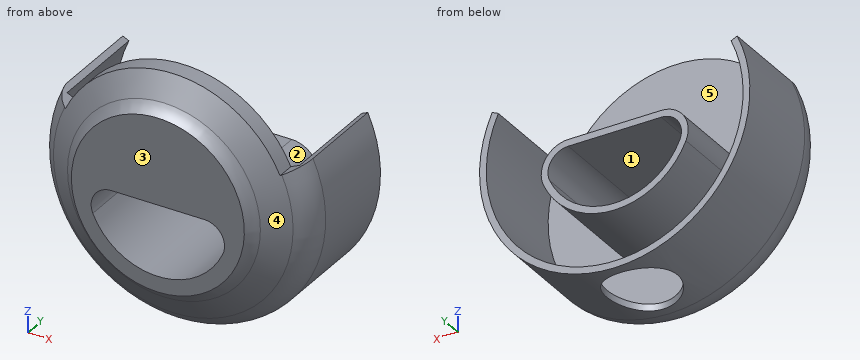
from build123d import *

# Parameters (mm, degrees)
CUT_EXTRUDE3_DEPTH           = 60
CUT_EXTRUDE5_DEPTH           = 2
CUT_EXTRUDE5_DEPTH_BACK      = 30
SKETCH9_R                    = 38
SKETCH9_R_2                  = 23
SKETCH19_W                   = 12
SKETCH19_H                   = 36.5
CUT_REVOLVE2_ANGLE           = 65
CUT_REVOLVE2_OTHER_WAY_ANGLE = 65
SKETCH21_W                   = 3.25
SKETCH21_H                   = 4
BOSS_EXTRUDE3_DEPTH          = 1.35
CIRPATTERN1_COUNT            = 5
CUT_EXTRUDE9_START           = -5
CUT_EXTRUDE9_DEPTH           = 5
SKETCH23_R                   = 10.5
CUT_EXTRUDE10_DEPTH          = 10
SKETCH24_W                   = 15
SKETCH24_H                   = 8
BOSS_EXTRUDE4_DEPTH          = 8
SKETCH26_W                   = 10
SKETCH26_H                   = 6
CUT_EXTRUDE11_DEPTH          = 10
SKETCH27_W                   = 4
SKETCH27_H                   = 5
CUT_EXTRUDE12_DEPTH          = 5
CUT_EXTRUDE14_DEPTH          = 2
CUT_EXTRUDE14_DEPTH_BACK     = 30
SKETCH29_R                   = 1
CUT_EXTRUDE15_DEPTH          = 15
FILLET1_R                    = 6
FILLET2_R                    = 8
INTERSECT2_START             = 55.427876097
INTERSECT2_OUTLINE_W         = 10
INTERSECT2_OUTLINE_H         = 6
INTERSECT2_DEPTH             = 8
INTERSECT2_2_DEPTH           = 13
INTERSECT2_START_2           = 50.427876097
INTERSECT2_3_OUTLINE_W       = 15
INTERSECT2_3_OUTLINE_H       = 8
INTERSECT2_3_OUTLINE_W_2     = 10
INTERSECT2_3_OUTLINE_H_2     = 6
INTERSECT2_3_DEPTH           = 5


# Read off the part's stored shape, not the designer's step: Cut-Extrude9, Intersect2
with BuildPart() as part:
    # Sketch1 → Revolve1 (revolve)
    with BuildSketch(Plane.XY, mode=Mode.PRIVATE) as revolve1_sk:
        with BuildLine():
            Line((0, 63.427876097), (32, 63.427876097))
            ThreePointArc((32, 63.427876097), (37.656854249, 61.084730346), (40, 55.427876097))
            Line((40, 55.427876097), (40, 28.846818009))
            ThreePointArc((40, 28.846818009), (38.792081772, 24.082439968), (35.460140376, 20.469057744))
            Line((35.460140376, 20.469057744), (28.539859624, 15.958818353))
            ThreePointArc((28.539859624, 15.958818353), (25.207918228, 12.345436129), (24, 7.581058088))
            Line((24, 7.581058088), (24, 3.25))
            Line((24, 3.25), (24.35, 3))
            Line((24.35, 3), (24.35, 0))
            Line((24.35, 0), (22.5, 0))
            Line((22.5, 0), (22.5, 12.5))
            ThreePointArc((22.5, 12.5), (22.353553391, 12.853553391), (22, 13))
            Line((22, 13), (0, 13))
            Line((0, 13), (0, 63.427876097))
        make_face()
    revolve(revolve1_sk.sketch.rotate(Axis((0, 0, 0), (0, 1, 0)), 90), axis=Axis((0, 0, 0), (0, 1, 0)))

    # Sketch11 → Cut-Extrude3 (cut)
    with BuildSketch(Plane(origin=(0, 13, 0), x_dir=(-1, 0, 0), z_dir=(0, -1, 0))):
        with BuildLine():
            Line((-21, 0), (21, 0))
            ThreePointArc((21, 0), (0, 21), (-21, 0))
        make_face()
    extrude(amount=-CUT_EXTRUDE3_DEPTH, mode=Mode.SUBTRACT)

    # Sketch9 → Cut-Extrude5 (cut, two sides: drawn at the far end of the back side and taken through both)
    with BuildSketch(Plane(origin=(0, 55.427876097, 0), x_dir=(1, 0, 0), z_dir=(0, 1, 0)).offset(-CUT_EXTRUDE5_DEPTH_BACK)):
        with Locations(Location((0, 0, 0), (0, 0, 270))):
            Circle(SKETCH9_R)
        with Locations(Location((0, 0, 0), (0, 0, 270))):
            Circle(SKETCH9_R_2, mode=Mode.SUBTRACT)
    extrude(amount=CUT_EXTRUDE5_DEPTH + CUT_EXTRUDE5_DEPTH_BACK, mode=Mode.SUBTRACT)

    # Sketch19 → Cut-Revolve2 (revolve, cut)
    with BuildSketch(Plane(origin=(0, 0, 0), x_dir=(0, 0, -1), z_dir=(1, 0, 0))):
        with Locations((-41.064715832, 37.177876097)):
            Rectangle(SKETCH19_W, SKETCH19_H)
    revolve(axis=Axis((0, 0, 0), (0, 1, 0)), revolution_arc=CUT_REVOLVE2_ANGLE, mode=Mode.SUBTRACT)

    # Sketch19 → Cut-Revolve2 other way (revolve, cut)
    with BuildSketch(Plane(origin=(0, 0, 0), x_dir=(0, 0, -1), z_dir=(1, 0, 0))):
        with Locations((-41.064715832, 37.177876097)):
            Rectangle(SKETCH19_W, SKETCH19_H)
    revolve(axis=Axis((0, 0, 0), (0, -1, 0)), revolution_arc=CUT_REVOLVE2_OTHER_WAY_ANGLE, mode=Mode.SUBTRACT)

    # Sketch21 → Boss-Extrude3 (add)
    with BuildSketch(Plane(origin=(0, 0, 22.5), x_dir=(-1, 0, 0), z_dir=(0, 0, -1))):
        with Locations((0, 2)):
            Rectangle(SKETCH21_W, SKETCH21_H)
    boss_extrude3 = extrude(amount=BOSS_EXTRUDE3_DEPTH)

    # CirPattern1: Boss-Extrude3 ×5 about axis
    cirpattern1_axis = Axis((0, 0, 0), (0, 1, 0))
    for i in range(1, CIRPATTERN1_COUNT):
        add(boss_extrude3.rotate(cirpattern1_axis, i * 360 / CIRPATTERN1_COUNT))

    # Cut-Extrude9 outline → Cut-Extrude9 (cut)
    with BuildSketch(Plane(origin=(0, 63.427876097, 0), x_dir=(1, 0, 0), z_dir=(0, 1, 0)).offset(CUT_EXTRUDE9_START)):
        with BuildLine():
            ThreePointArc((40, 0), (0, 40), (-40, 0))
            Line((-40, 0), (-21, 0))
            ThreePointArc((-21, 0), (0, 21), (21, 0))
            Line((21, 0), (40, 0))
        make_face()
    extrude(amount=CUT_EXTRUDE9_DEPTH, mode=Mode.SUBTRACT)

    # Sketch23 → Cut-Extrude10 (cut)
    with BuildSketch(Plane(origin=(0, 0, -40), x_dir=(-1, 0, 0), z_dir=(0, 0, -1))):
        with Locations((0, 42.137876097)):
            Circle(SKETCH23_R)
    extrude(amount=-CUT_EXTRUDE10_DEPTH, mode=Mode.SUBTRACT)

    # Sketch24 → Boss-Extrude4 (add)
    with BuildSketch(Plane(origin=(0, 58.427876097, 0), x_dir=(1, 0, 0), z_dir=(0, 1, 0))):
        with Locations((0, 30)):
            Rectangle(SKETCH24_W, SKETCH24_H)
    extrude(amount=-BOSS_EXTRUDE4_DEPTH)

    # Sketch26 → Cut-Extrude11 (cut)
    with BuildSketch(Plane(origin=(0, 58.427876097, 0), x_dir=(1, 0, 0), z_dir=(0, 1, 0))):
        with Locations((0, 30)):
            Rectangle(SKETCH26_W, SKETCH26_H)
    extrude(amount=-CUT_EXTRUDE11_DEPTH, mode=Mode.SUBTRACT)

    # Sketch27 → Cut-Extrude12 (cut)
    with BuildSketch(Plane(origin=(7.5, 0, 0), x_dir=(0, 0, -1), z_dir=(1, 0, 0))):
        with Locations((30, 53.927876097)):
            Rectangle(SKETCH27_W, SKETCH27_H)
    extrude(amount=-CUT_EXTRUDE12_DEPTH, mode=Mode.SUBTRACT)

    # Sketch28 → Cut-Extrude14 (cut, two sides: drawn at the far end of the back side and taken through both)
    with BuildSketch(Plane(origin=(0, 55.427876097, 0), x_dir=(1, 0, 0), z_dir=(0, 1, 0)).offset(-CUT_EXTRUDE14_DEPTH_BACK)):
        with BuildLine():
            Line((-22.912878475, -2), (22.912878475, -2))
            ThreePointArc((22.912878475, -2), (0, -23), (-22.912878475, -2))
        make_face()
    extrude(amount=CUT_EXTRUDE14_DEPTH + CUT_EXTRUDE14_DEPTH_BACK, mode=Mode.SUBTRACT)

    # Sketch29 → Cut-Extrude15 (cut)
    with BuildSketch(Plane(origin=(0, 0, 0), x_dir=(-1, 0, 0), z_dir=(0, 0, -1))):
        with Locations((-30.416198487, 60.927876097)):
            Circle(SKETCH29_R)
        with Locations((30.416198487, 60.927876097)):
            Circle(SKETCH29_R)
        with Locations((0, 60.927876097)):
            Circle(SKETCH29_R)
    extrude(amount=-CUT_EXTRUDE15_DEPTH, mode=Mode.SUBTRACT)

    # Fillet1
    fillet1_edges = [part.edges().sort_by_distance(p)[0] for p in [
        (21, 35.713938048, 0),
        (-21, 35.713938048, 0),
    ]]
    fillet(fillet1_edges, radius=FILLET1_R)

    # Fillet2
    fillet2_edges = [part.edges().sort_by_distance(p)[0] for p in [
        (-22.912878475, 41.427876097, 2),
        (22.912878475, 41.427876097, 2),
    ]]
    fillet(fillet2_edges, radius=FILLET2_R)

    # Intersect2 outline → Intersect2 (cut)
    with BuildSketch(Plane(origin=(0, 0, 0), x_dir=(1, 0, 0), z_dir=(0, 1, 0)).offset(INTERSECT2_START)):
        Polygon((-42, -15), (-40.906642577, -15), (-42, -15.355253362), (-42, -42), (42, -42), (42, -15.355253362), (40.906642577, -15), (42, -15), (42, 32), (25.257971351, 32), (32.523396625, 42), (-32.523396625, 42), (-25.257971351, 32), (-42, 32), align=None)
        with Locations((0, 30)):
            Rectangle(INTERSECT2_OUTLINE_W, INTERSECT2_OUTLINE_H, mode=Mode.SUBTRACT)
    extrude(amount=INTERSECT2_DEPTH, mode=Mode.SUBTRACT)

    # Intersect2 2 outline → Intersect2 2 (cut)
    with BuildSketch(Plane(origin=(0, 0, 0), x_dir=(1, 0, 0), z_dir=(0, 1, 0))):
        Polygon((-42, 28), (-42, -15), (-40.906642577, -15), (-42, -15.355253362), (-42, -42), (42, -42), (42, -15.355253362), (40.906642577, -15), (42, -15), (42, 28), (7.5, 28), (7.5, 26), (-7.5, 26), (-7.5, 28), align=None)
    extrude(amount=INTERSECT2_2_DEPTH, mode=Mode.SUBTRACT)

    # Intersect2 3 outline → Intersect2 3 (cut)
    with BuildSketch(Plane(origin=(0, 0, 0), x_dir=(1, 0, 0), z_dir=(0, 1, 0)).offset(INTERSECT2_START_2)):
        with Locations((0, 30)):
            Rectangle(INTERSECT2_3_OUTLINE_W, INTERSECT2_3_OUTLINE_H)
        with Locations((0, 30)):
            Rectangle(INTERSECT2_3_OUTLINE_W_2, INTERSECT2_3_OUTLINE_H_2, mode=Mode.SUBTRACT)
    extrude(amount=INTERSECT2_3_DEPTH, mode=Mode.SUBTRACT)


solid = part.part
Geometry check sheet. Reference: the model listing, model coordinates, mm. Face numbers are marked on the shaded views. A direction names the side the tool comes from. Round coordinates to 2 decimals unless told otherwise and drop trailing zeros. Write each loop counter-clockwise with the first axis right and the second up, starting at its lowest first coordinate (ties: lowest second). Pieces come first, ordered by that corner, then holes. Notation, with made-up numbers: (40.25, 41) -> (61.25, 41) arc R20 cw to (61.25, 68) -> close; hole circle Ø3 at (77.25, -12.75). An arc over 180 degrees is marked (long way). One line per item, written item: value. Start each with the question number.
(1) Go/stop test with flat-tipped pins: pin 1 Ø8 at (x, y) = (-23, 19) entering from -Z; pin 2 Ø5 at (x, y) = (-30.5, 36) entering from +Z; pin 3 Ø1 at (x, y) = (-17.5, 34) entering from -Z. Record where each tip stops, or that it passes through.
(2) Draft check along Z on the marked faces 3, 4 and 5. Enter one of: +Z half, -Z half, draft (parallel to the pull), parting line (faces both ways), or undercut.
(3) Cross-section at C-C, the plane x = -9. Give the number of separate pieces and of enclosed holes in the cut face, and give its area (3 significant figures).
(4) Cross-section at B-B, the plane x = 0. Record the cut outline in (y, z), and give its area (3 significant figures).
(5) Scan lines: line 1 (Z direction, x = 7, y = 26.5); line 2 (Z direction, x = 0, y = 44.5); line 3 (X direction, y = 48.5, z = -6). Record each from-to range of solid material in increasing order. Write a range as [from, to].
(6) Access from +Z, -Z, +X, -X, +Y, -Y to the whole of each face (thin tool, end or side, straight path). Record for the marked faces 1 and 2.
(7) Cross-section at A-A, the plane y = 26.5. Record the cut outline in (x, z), and give its area (3 significant figures).
Answer:
1. pin 1: z = -31.32
1. pin 2: z = -18.84
1. pin 3: z = -36.21
2. face 3: draft
2. face 4: parting line
2. face 5: undercut
3. separate pieces: 3
3. enclosed holes: 0
3. area: 706 mm²
4. outline: (13, -25.6) arc R10 cw to (15.96, -28.54) -> (20.47, -35.46) arc R10 ccw to (28.85, -40) -> (31.64, -40) -> (31.64, -38) -> (25.43, -38) -> (25.43, -23) -> (55.43, -23) -> (55.43, -21) -> (13, -21) -> close; (13, 0) -> (55.43, 0) -> (55.43, 2) -> (25.43, 2) -> (25.43, 35.06) -> (20.21, 35.06) -> (15.96, 28.54) arc R10 cw to (13, 25.6) -> close; (52.64, -40) -> (55.43, -40) -> (55.43, -38) -> (52.64, -38) -> close
4. area: 686 mm²
5. line 1: [-39.1, -37.35], [-21.91, -19.8], [0, 2]
5. line 2: [-23, -21], [0, 2]
5. line 3: [-39.55, -37.52], [-21.75, -19.75], [19.75, 21.75], [37.52, 39.55]
6. face 1: +Y, -Y
6. face 2: +Y
7. outline: (-36, 16.79) arc R39.72 ccw (long way) to (36, 16.79) -> (34.44, 16.06) arc R38 cw (long way) to (-34.44, 16.06) -> close; (-21.08, -9.2) arc R23 ccw to (21.08, -9.2) arc R8 ccw to (13.75, 2) -> (-13.75, 2) arc R8 ccw to start; hole (-19.25, -8.4) arc R21 ccw to (19.25, -8.4) arc R6 ccw to (13.75, 0) -> (-13.75, 0) arc R6 ccw to start
7. area: 481 mm²
